Autodesk Inventor part; units mm, degrees
ref_plane "YZ Plane" through (0, 0, 0) normal (1, 0, 0) x (0, 1, 0)
ref_plane "XZ Plane" through (0, 0, 0) normal (0, 1, 0) x (-1, 0, 0)
ref_plane "XY Plane" through (0, 0, 0) normal (0, 0, 1) x (1, 0, 0)
sketch "Sketch1" plane through (0, 0, 0) normal (0, 0, 1) x (1, 0, 0)
  line L0 (12.7, -6.0198) -> (-12.7, -6.0198)
  line L1 (-12.7, -6.0198) -> (-12.7, 6.0198)
  line L2 (-12.7, 6.0198) -> (12.7, 6.0198)
  line L3 (12.7, 6.0198) -> (12.7, -6.0198)
  line L4 (12.7, -6.0198) -> (-12.7, 6.0198) construction
  line L5 (-12.7, -6.0198) -> (12.7, 6.0198) construction
  point P0 (0, 0)
  dimension "d0" = 25.4
  dimension "d1" = 12.0396
extrude "Extrusion1" add sketch "Sketch1" along normal blind 31.75
shell "Shell1" thickness 2.54 removed faces 2 at (4.2333, -2.0066, 0) at (4.2333, -2.0066, 31.75)
sketch "Sketch2" plane through (-12.7, 6.0198, 0) normal (0, 1, 0) x (1, 0, 0)
  line L0 (-2.1226, -3.175) -> (30.0619, -3.175)
  line L1 (0, 0) -> (25.4, 0)
  circle A0 centre (7.874, -3.175) radius 1.524
  circle A1 centre (17.526, -3.175) radius 1.524
  line L2 (12.7, 1.1779) -> (12.7, -16.2415)
  point P0 (12.7, 0)
  point P1 (12.7, 0)
  dimension "d23" = 3.175
  dimension "d24" = 3.048
  dimension "d25" = 9.652
extrude "Extrusion2" cut sketch "Sketch2" against normal through all
sketch "Sketch3" plane through (0, 0, 31.75) normal (0, 0, 1) x (1, 0, 0)
  line L0 (-10.16, 3.4798) -> (10.16, 3.4798)
  line L1 (10.16, 3.4798) -> (10.16, -3.4798)
  line L2 (10.16, -3.4798) -> (-10.16, -3.4798)
  line L3 (-10.16, -3.4798) -> (-10.16, 3.4798)
  line L4 (-10.16, 3.4798) -> (10.16, -3.4798) construction
  line L5 (10.16, 3.4798) -> (-10.16, -3.4798) construction
  line L6 (-12.7, 9.525) -> (12.7, 9.525)
  line L7 (15.875, 6.35) -> (15.875, -6.35)
  line L8 (12.7, -9.525) -> (-12.7, -9.525)
  line L9 (-15.875, -6.35) -> (-15.875, 6.35)
  line L10 (-15.875, 9.525) -> (15.875, -9.525) construction
  line L11 (15.875, 9.525) -> (-15.875, -9.525) construction
  arc A0 (12.7, -9.525) -> (15.875, -6.35) centre (12.7, -6.35) ccw
  arc A1 (15.875, 6.35) -> (12.7, 9.525) centre (12.7, 6.35) ccw
  arc A2 (-12.7, 9.525) -> (-15.875, 6.35) centre (-12.7, 6.35) ccw
  arc A3 (-15.875, -6.35) -> (-12.7, -9.525) centre (-12.7, -6.35) ccw
  point P0 (0, 0)
  dimension "d28" = 19.05
  dimension "d29" = 31.75
  dimension "d30" = 3.175
extrude "Extrusion3" add sketch "Sketch3" along normal blind 3.175
fillet "Fillet1" radius 3.175 4 edges at (12.7, 6.0198, 15.875) (12.7, -6.0198, 15.875) (-12.7, 6.0198, 15.875) (-12.7, -6.0198, 15.875)
properties part number "E-Stop_Fixture_Taller"
Input: part model. Units: mm. Frame: model coordinates. A direction names the side the tool comes from. Coordinates: 2 decimals unless noted, no trailing zeros. Loops run counter-clockwise (first coordinate to the right, second up) from the corner with the lowest first, then second, coordinate; pieces in that order, holes last. Notation, with made-up numbers: (26.25, -25.75) -> (32.25, -25.75) arc R6 cw to (32.25, -17.75) -> close; hole circle Ø5 at (27.25, 41). An arc over 180 degrees is marked (long way). One line per item, written item: value.
(1) Set-up query: faces 1 (the face through (11.75, -5.11, 16.1)), 2 (the face through (0, 6.02, 16)), 3 (the face through (0, -3.48, 17)), 4 (the face through (12.7, 0, 16)). Return all of +Z, -Z, +X, -X, +Y, -Y with unobstructed straight access to the full face (end or side cutting, diameter ignored); none if empty.
Answer below:
face 1: -Z, +X, -Y
face 2: -Z, +X, -X, +Y
face 3: +Z, -Z
face 4: -Z, +X, +Y, -Y
(2) Draft query along Y for faces 5 (the face through (14.97, -8.57, 33.32)), 6 (the face through (-6.35, -4.73, 3.11)), 7 (the face through (10.16, 0, 17)). Return one class per face: pulls with the +Y half, pulls with the -Y half, needs draft (parallel to the pull), parting line crosses it, or undercut.
Answer below:
face 5: pulls with the -Y half
face 6: needs draft
face 7: undercut
(3) Ray query, line 1 along Y through (x, z) = (-4, 23.5); line 2 along X through (y, z) = (2, 18); line 3 along Z through (x, y) = (-5, -7.5) (3 decimals). Return the intervals inside material, ascending.
Answer below:
line 1: y = -6.02 to -3.48, 3.48 to 6.02
line 2: x = -12.7 to -10.16, 10.16 to 12.7
line 3: z = 31.75 to 34.925
(4) Cut plane B-B (y = -2.25). Output: boundary loops of the cut face in (x, z) (3 decimals).
Answer below:
outline: (-15.875, 31.75) -> (-12.7, 31.75) -> (-12.7, 0) -> (-10.16, 0) -> (-10.16, 34.925) -> (-15.875, 34.925) -> close; (10.16, 0) -> (12.7, 0) -> (12.7, 31.75) -> (15.875, 31.75) -> (15.875, 34.925) -> (10.16, 34.925) -> close
(5) Pin query (flat end, axial travel): pin 1 Ø3.5 at (x, z) = (-4.826, 3.175) entering from -Y; pin 2 Ø8 at (y, z) = (3, 26) entering from +X; pin 3 Ø1.7 at (y, z) = (0.5, 13) entering from -X. Return the tip coordinate at first contact, or that it passes through.
Answer below:
pin 1: stops at y = -6.02
pin 2: stops at x = 12.7
pin 3: stops at x = -12.7
(6) Cut plane A-A (x = 8.5). Output: boundary loops of the cut face in (y, z) (3 decimals), then the cut area to 3 significant figures.
Answer below:
outline: (-9.525, 31.75) -> (-6.02, 31.75) -> (-6.02, 0) -> (-3.48, 0) -> (-3.48, 34.925) -> (-9.525, 34.925) -> close; (3.48, 0) -> (6.02, 0) -> (6.02, 31.75) -> (9.525, 31.75) -> (9.525, 34.925) -> (3.48, 34.925) -> close
area: 200 mm2
(7) Cut plane C-C (z = 21). Output: boundary loops of the cut face in (x, y) (3 decimals), then the cut area to 3 significant figures.
Answer below:
outline: (-12.7, -2.845) arc R3.175 ccw to (-9.525, -6.02) -> (9.525, -6.02) arc R3.175 ccw to (12.7, -2.845) -> (12.7, 2.845) arc R3.175 ccw to (9.525, 6.02) -> (-9.525, 6.02) arc R3.175 ccw to (-12.7, 2.845) -> close; hole (-10.16, -3.48) -> (10.16, -3.48) -> (10.16, 3.48) -> (-10.16, 3.48) -> close
area: 156 mm2
(8) Cut plane D-D (y = 5.25). Output: boundary loops of the cut face in (x, z) (3 decimals).
Answer below:
outline: (-15.875, 31.75) -> (-11.598, 31.75) -> (-11.598, 0) -> (11.598, 0) -> (11.598, 31.75) -> (15.875, 31.75) -> (15.875, 34.925) -> (-15.875, 34.925) -> close; hole circle Ø3.048 at (-4.826, 3.175); hole circle Ø3.048 at (4.826, 3.175)
